The listing builds one solid part. Answer for the finished solid, in the listing's coordinates (mm). Give positions to 0.01 mm unless a question says otherwise; leave off trailing zeros. Answer in a Markdown table with one row per item. Add a question column.
from build123d import *

# Parameters (mm, degrees)
F0_R     = 2.1
F1_DEPTH = 300


with BuildPart() as f1:
    # F0 (on Front) → F1 (new body)
    with BuildSketch(Plane.XZ):
        with BuildLine():
            Line((4.585786, 6), (0, 6))
            Line((0, 6), (-4.585786, 6))
            Line((-4.585786, 6), (-8.25, 9.664214))
            Line((-8.25, 9.664214), (-8.25, 13))
            Line((-8.25, 13), (-4, 13))
            Line((-4, 13), (-4, 15))
            Line((-4, 15), (-13, 15))
            ThreePointArc((-13, 15), (-14.414214, 14.414214), (-15, 13))
            Line((-15, 13), (-15, 4))
            Line((-15, 4), (-13, 4))
            Line((-13, 4), (-13, 8.25))
            Line((-13, 8.25), (-9.664214, 8.25))
            Line((-9.664214, 8.25), (-6, 4.585786))
            Line((-6, 4.585786), (-6, 0))
            Line((-6, 0), (-6, -4.585786))
            Line((-6, -4.585786), (-9.664214, -8.25))
            Line((-9.664214, -8.25), (-13, -8.25))
            Line((-13, -8.25), (-13, -4))
            Line((-13, -4), (-15, -4))
            Line((-15, -4), (-15, -13))
            ThreePointArc((-15, -13), (-14.414214, -14.414214), (-13, -15))
            Line((-13, -15), (-4, -15))
            Line((-4, -15), (-4, -13))
            Line((-4, -13), (-8.25, -13))
            Line((-8.25, -13), (-8.25, -9.664214))
            Line((-8.25, -9.664214), (-4.585786, -6))
            Line((-4.585786, -6), (0, -6))
            Line((0, -6), (4.585786, -6))
            Line((4.585786, -6), (8.25, -9.664214))
            Line((8.25, -9.664214), (8.25, -13))
            Line((8.25, -13), (4, -13))
            Line((4, -13), (4, -15))
            Line((4, -15), (13, -15))
            ThreePointArc((13, -15), (14.414214, -14.414214), (15, -13))
            Line((15, -13), (15, -4))
            Line((15, -4), (13, -4))
            Line((13, -4), (13, -8.25))
            Line((13, -8.25), (9.664214, -8.25))
            Line((9.664214, -8.25), (6, -4.585786))
            Line((6, -4.585786), (6, 0))
            Line((6, 0), (6, 4.585786))
            Line((6, 4.585786), (9.664214, 8.25))
            Line((9.664214, 8.25), (13, 8.25))
            Line((13, 8.25), (13, 4))
            Line((13, 4), (15, 4))
            Line((15, 4), (15, 13))
            ThreePointArc((15, 13), (14.414214, 14.414214), (13, 15))
            Line((13, 15), (4, 15))
            Line((4, 15), (4, 13))
            Line((4, 13), (8.25, 13))
            Line((8.25, 13), (8.25, 9.664214))
            Line((8.25, 9.664214), (4.585786, 6))
        make_face()
        with Locations((-11.6, -11.6)):
            Circle(F0_R, mode=Mode.SUBTRACT)
        with Locations((11.6, -11.6)):
            Circle(F0_R, mode=Mode.SUBTRACT)
        with Locations((-11.6, 11.6)):
            Circle(F0_R, mode=Mode.SUBTRACT)
        with BuildLine():
            ThreePointArc((-3.4, 0), (-2.404163, 2.404163), (0, 3.4))
            ThreePointArc((0, 3.4), (2.404163, 2.404163), (3.4, 0))
            ThreePointArc((3.4, 0), (2.404163, -2.404163), (0, -3.4))
            ThreePointArc((0, -3.4), (-2.404163, -2.404163), (-3.4, 0))
        make_face(mode=Mode.SUBTRACT)
        with Locations((11.6, 11.6)):
            Circle(F0_R, mode=Mode.SUBTRACT)
    extrude(amount=F1_DEPTH)


solid = f1.part
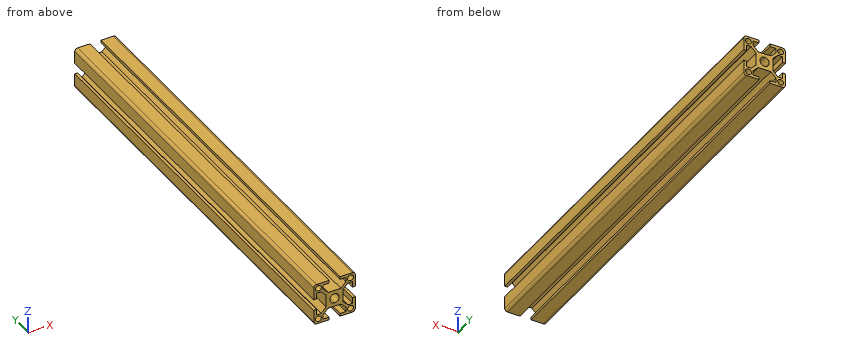
1. Given pin 1 Ø2 at (x, y) = (-14.5, -104.5) entering from +Z; pin 2 Ø1.6 at (y, z) = (-145.5, -14) entering from +X, each flat-ended and moving along its own axis, determine where each tip first touches the part or whether it passes through.
2. Section A-A (y = -24.5) is taken. State how many separate pieces and enclosed holes the cut face has, and give its area (3 significant figures).
3. Straight lines are drawn through the part: L1, parallel to Z at x = -12, y = -157.5; L2, parallel to X at y = -276, z = 10. For each, find the intervals that lie inside material, in ascending order. Write a range as [from, to].
Geometry check:
| question | item | result |
|---|---|---|
| 1 | pin 1 | z = 14.94 |
| 1 | pin 2 | x = 14.99 |
| 2 | separate pieces | 1 |
| 2 | enclosed holes | 5 |
| 2 | area | 333 mm² |
| 3 | L1 | [-15, -13.66], [-9.54, -8.25], [8.25, 9.54], [13.66, 15] |
| 3 | L2 | [-15, -12.96], [-10.24, -8.25], [8.25, 10.24], [12.96, 15] |
